CAD build for the part. Positions are in the model's coordinates, mm. Give positions to 0.01 mm unless a question says otherwise; leave off trailing zeros. Order: outer loops, then holes, each group sorted by start corner. A loop starts at its lowest first (then second) coordinate and runs counter-clockwise, first axis right, second up. Notation, with made-up numbers: (79, -3) -> (119, -3) arc R12 ccw to (119, 2) -> close; hole circle Ø7 at (41.25, -7.5). An arc over 180 degrees is marked (long way). Use one line per item in the form item = value. Start each with the question number.
1) Probe line 1 (Y direction, x = -6, z = 13); line 2 (X direction, y = 11, z = 14.5); line 3 (Y direction, x = -4, z = 18). List the from-to ranges inside material, lowest first.
2) Cut at A-A, the plane z = 14.5. Give the cut face in (x, y).
3) Drop flat-ended pins along their axis: P1, Ø4.5, axis at y = -12.5, z = 22, coming from the +X side; P2, Ø3, axis at y = -13, z = 22, coming from the -X side; P3, Ø6, axis at x = 12.5, y = -32.5, coming from the -Z side. Give the stop position or say it passes through.
from build123d import *

# Parameters (mm, degrees)
F1_ANGLE_BACK = 90
F1_ANGLE      = 180
F2_W          = 19.5003319532
F2_H          = 42.3330869526
F3_DEPTH      = 15.24
F2_W_2        = 6.9107273594
F2_H_2        = 20.5113845763
F4_DEPTH      = 6.35
F5_SIZE       = 6.35
F6_SIZE       = 6.223
F7_W          = 3.429
F7_H          = 5.08
F8_DEPTH      = 0.508


with BuildPart() as f1:
    # F0 (on Right) → F1 (revolve)
    with BuildSketch(Plane.YZ, mode=Mode.PRIVATE) as f1_sk:
        with BuildLine():
            Line((34.9214076996, 10.6095829979), (-70.8683729172, 10.9261889011))
            add(Edge.make_bspline(
                [(-70.8683729172, 10.9261889011), (-70.1419854561, 10.2578587346), (-68.0454930222, 7.6017228607), (-46.8309506702, -4.8443860401), (-23.6054190841, -6.038263541), (-7.9588431838, -5.7330571075), (19.1368285034, -5.8978473622), (28.0721145699, -5.7025676976), (32.1389431313, -2.954042184), (34.975613757, 4.252374343), (35.0640308282, 6.9227486413), (34.9214076996, 10.6095829979)],
                knots=[0, 0, 0, 0, 0.0622616351, 0.2180374171, 0.3738682141, 0.5047076416, 0.6710416497, 0.7649499794, 0.8315827282, 0.9148966955, 1, 1, 1, 1], degree=3))
        make_face()
    revolve(f1_sk.sketch.rotate(Axis((0, -17.9734826088, 10.7678859495), (0, -0.9999955217, 0.00299277)), -F1_ANGLE_BACK), axis=Axis((0, -17.9734826088, 10.7678859495), (0, -0.9999955217, 0.00299277)), revolution_arc=F1_ANGLE)

    # F2 (on face) → F3 (join)
    with BuildSketch(Plane(origin=(0, 0.0320646795, 10.7139992458), x_dir=(1, 0, 0), z_dir=(0, 0.00299277, 0.9999955217))):
        with Locations((0, 5.5756000802)):
            Rectangle(F2_W, F2_H)
    extrude(amount=F3_DEPTH)

    # F2 (on face) → F4 (join)
    with BuildSketch(Plane(origin=(0, 0.0320646795, 10.7139992458), x_dir=(1, 0, 0), z_dir=(0, 0.00299277, 0.9999955217))):
        with Locations((0, -40.5601523817)):
            Rectangle(F2_W_2, F2_H_2)
    extrude(amount=F4_DEPTH)

    # F5
    f5_edges = [f1.edges().sort_by_distance(p)[0] for p in [
        (0, -15.513199, 26.000591),
    ]]
    chamfer(f5_edges, length=F5_SIZE)

    # F6
    f6_edges = [f1.edges().sort_by_distance(p)[0] for p in [
        (0, -50.764548, 17.216051),
    ]]
    chamfer(f6_edges, length=F6_SIZE)

    # F7 (on face) → F8 (cut)
    with BuildSketch(Plane(origin=(0, -17.5447512472, 17.6500817605), x_dir=(1, 0, 0), z_dir=(0, -0.7049874065, 0.7092198225))):
        with Locations((0, 7.2997931698)):
            Rectangle(F7_W, F7_H)
        with Locations((6.604, 7.327820993)):
            Rectangle(F7_W, F7_H)
        with Locations((-6.604, 7.327820993)):
            Rectangle(F7_W, F7_H)
    extrude(amount=-F8_DEPTH, mode=Mode.SUBTRACT)


solid = f1.part
Result:
q1.line_1 = -15.55 to 26.78
q1.line_2 = -9.75 to 9.75
q1.line_3 = -15.54 to 26.8
q2.outline = (-9.75, -15.55) -> (9.75, -15.55) -> (9.75, 26.79) -> (-9.75, 26.79) -> close; (-3.46, -47.26) -> (3.46, -47.26) -> (3.46, -30.26) -> (-3.46, -30.26) -> close
q3.P1 = 9.75
q3.P2 = -9.75
q3.P3 = -2.33
